Work out the finished part from the listing and answer in its coordinate system (mm). Face numbers are marked on the shaded views. Coordinates: 2 decimals unless noted, no trailing zeros. Order: outer loops, then holes, each group sorted by start corner. A loop starts at its lowest first (then second) coordinate and runs counter-clockwise, first axis right, second up. Notation, with made-up numbers: (-21.75, 66.5) -> (8.25, 66.5) arc R21 ccw to (8.25, 91.5) -> close; hole circle Ø6 at (29, -26). An arc over 180 degrees is marked (long way). Write item = value, one per line. Start each with the question number.
Q1. Flat-ended cylindrical pins translate along their axes: pin 1 (6 mm diameter, centred on y = 180, z = -35, fed in from -X); pin 2 (8 mm diameter, centred on y = 3.5, z = -15.5, fed in from +X); pin 3 (3 mm diameter, centred on x = 11, z = -17.5, fed in from +Y). Find the tip coordinate at first contact, or state that the pin passes through.
Q2. The part is cut by section B-B, the plane z = -16.5. Determine the outline of the cut face in (x, y), plus the area to 3 significant figures.
Q3. The part is cut by section A-A, the plane x = 7.25. Determine the outline of the cut face in (y, z), plus the area to 3 significant figures.
Q4. The part is cut by section C-C, the plane y = 57. Determine the outline of the cut face in (x, z), plus the area to 3 significant figures.
Q5. Straight lines are drawn through the part: L1, parallel to Y at x = 6.25, z = -13; L2, parallel to X at y = 24, z = -16.5; L3, parallel to Y at x = 3.5, z = -31.5. For each, find the intervals that lie inside material, in ascending order. Write a range as from..to.
Q6. For a pull along Y with two mould halves and no side action, classify the marked faces 1 and 2 as +Y half, -Y half, draft (parallel to the pull), parting line (faces both ways), or undercut.
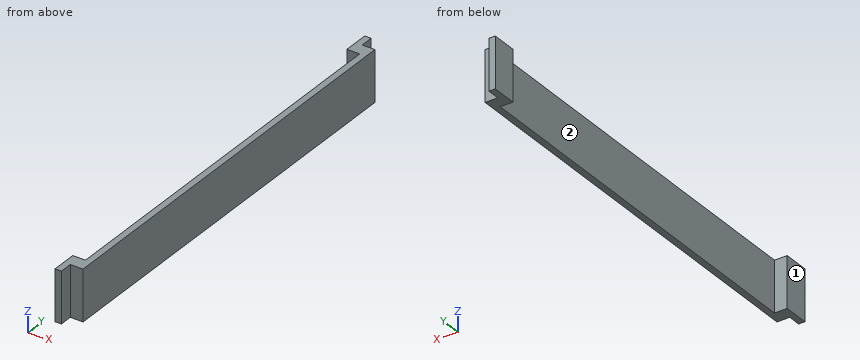
Autodesk Inventor part; units mm, degrees
ref_plane "YZ Plane" through (0, 0, 0) normal (1, 0, 0) x (0, 1, 0)
ref_plane "XZ Plane" through (0, 0, 0) normal (0, 1, 0) x (-1, 0, 0)
ref_plane "XY Plane" through (0, 0, 0) normal (0, 0, 1) x (1, 0, 0)
sketch "스케치1" plane through (0, 0, 0) normal (1, 0, 0) x (0, 1, 0)
  line L0 (0, 0) -> (20, 0)
  line L1 (20, 0) -> (20, -40)
  line L2 (20, -40) -> (0, -40)
  line L3 (0, -40) -> (0, 0)
  dimension "d0" = 20
  dimension "d1" = 40
extrude "돌출1" add sketch "스케치1" along normal blind 5
sketch "스케치2" plane through (5, 0, 0) normal (1, 0, 0) x (0, 0, -1)
  line L0 (40, 20) -> (0, 20)
  line L1 (0, 20) -> (40, 20)
  line L2 (40, 20) -> (40, 10)
  line L3 (40, 10) -> (0, 10)
  line L4 (0, 10) -> (0, 20)
  point P0 (0, 0)
  dimension "d4" = 40
  dimension "d5" = 10
extrude "돌출2" add sketch "스케치2" along normal blind 10
sketch "스케치3" plane through (15, 0, 0) normal (1, 0, 0) x (0, 0, -1)
  line L0 (0, 20) -> (40, 20)
  line L1 (40, 20) -> (40, 330)
  line L2 (40, 330) -> (0, 330)
  line L3 (0, 330) -> (0, 20)
  line L4 (40, 20) -> (0, 20)
  point P0 (0, 0)
  dimension "d8" = 40
  dimension "d9" = 310
extrude "돌출3" add sketch "스케치3" against normal blind 5
sketch "스케치4" plane through (15, 330, 0) normal (0, 1, 0) x (1, 0, 0)
  line L0 (0, 0) -> (0, 40)
  line L1 (-15, 40) -> (-15, 0)
  line L2 (0, 0) -> (-15, 0)
  line L3 (-15, 0) -> (-15, 40)
  line L4 (-15, 40) -> (0, 40)
  line L5 (0, 40) -> (0, 0)
  dimension "d15" = 15
  dimension "d16" = 40
extrude "돌출4" add sketch "스케치4" along normal blind 10
sketch "스케치5" plane through (15, 340, 0) normal (0, 1, 0) x (1, 0, 0)
  line L0 (-15, 40) -> (-10, 40)
  line L1 (-15, 40) -> (-10, 40)
  line L2 (-10, 40) -> (-10, 0)
  line L3 (-10, 0) -> (-15, 0)
  line L4 (-15, 0) -> (-15, 40)
  dimension "d19" = 5
  dimension "d20" = 40
extrude "돌출5" add sketch "스케치5" along normal blind 10
properties part number "link"
Model answer:
q1.pin_1 = 10
q1.pin_2 = 5
q1.pin_3 = 340
q2.outline = (0, 0) -> (5, 0) -> (5, 10) -> (15, 10) -> (15, 340) -> (5, 340) -> (5, 350) -> (0, 350) -> (0, 330) -> (10, 330) -> (10, 20) -> (0, 20) -> close
q2.area = 1,950 mm2
q3.outline = (10, -40) -> (20, -40) -> (20, 0) -> (10, 0) -> close; (330, -40) -> (340, -40) -> (340, 0) -> (330, 0) -> close
q3.area = 800 mm2
q4.outline = (10, -40) -> (15, -40) -> (15, 0) -> (10, 0) -> close
q4.area = 200 mm2
q5.L1 = 10..20, 330..340
q5.L2 = 10..15
q5.L3 = 0..20, 330..350
q6.face_1 = draft
q6.face_2 = undercut
